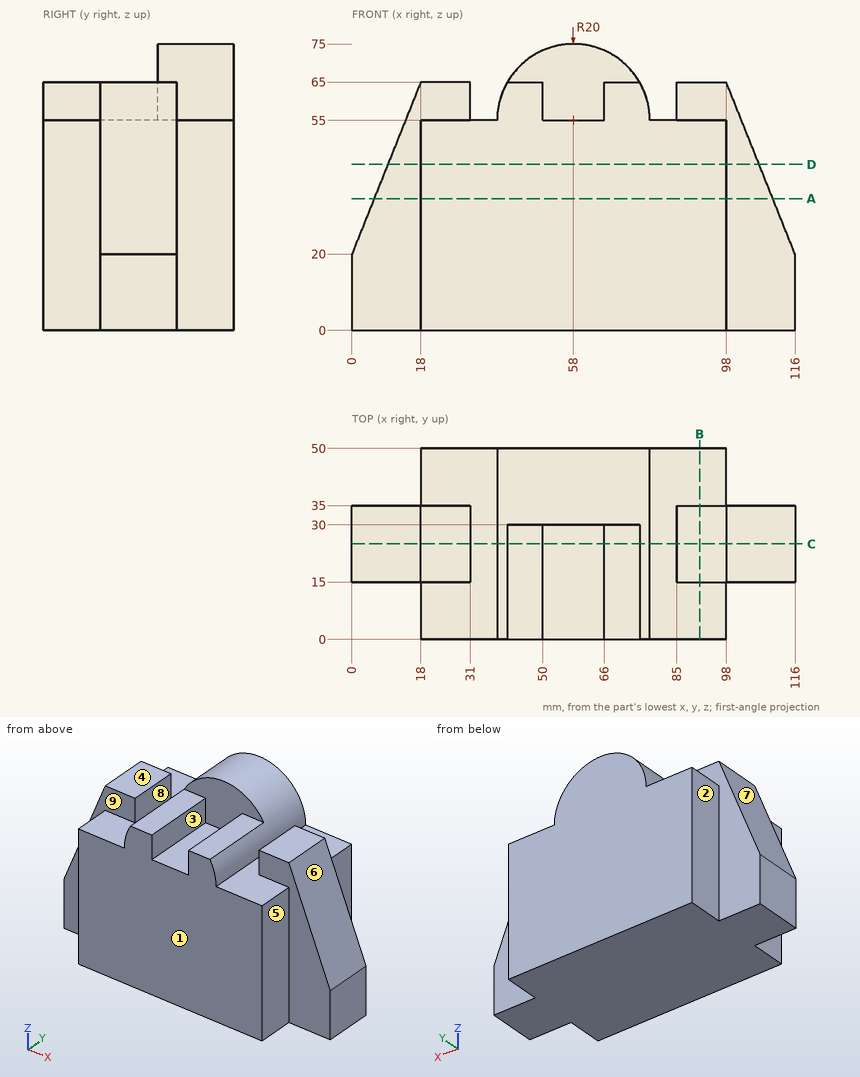
Could you check a few things on this drawing? It's one solid part, dimensions in mm from its lowest x, y, z. A direction names the side the tool comes from. Coordinates: 2 decimals unless noted, no trailing zeros. Write each loop counter-clockwise with the first axis right and the second up, starting at its lowest first coordinate (ties: lowest second). Pieces come first, ordered by that corner, then holes. Notation, with made-up numbers: (49.25, 31.25) - (67.25, 31.25) arc R8 ccw to (67.25, 41.25) - close; hole circle Ø7 at (89.5, 11). An arc over 180 degrees is marked (long way). Return JSON: item names as keys, results as strings. Group by question number.
Item 1: Which directions (+Z, -Z, +X, -X, +Y, -Y) give clear straight access to the entire face, cutting with the end or side of a thin tool? Please do the marked faces 1, 2, 3, 4 and 5.
Item 2: If we section it at B-B (x = 91): Write out the boundary of the cut face in (y, z), then the cut area to 3 significant figures.
Item 3: Please list where these lines run through material, in increasing order: probe 1 along X at (y, z) = (17.5, 64.5); probe 2 along X at (y, z) = (4, 32.5); probe 3 along Z at (x, y) = (56, 13.5).
Item 4: If we section it at D-D (z = 43.5): Write out the boundary of the cut face in (x, y), then the cut area to 3 significant figures.
Item 5: If we section it at A-A (z = 34.5): Write out the boundary of the cut face in (x, y).
Item 6: We'd pull the mould along X, two halves only. Please class the marked faces 6, 7, 8 and 9: pulls with the +X half, pulls with the -X half, needs draft (parallel to the pull), parting line crosses it, or undercut.
Item 7: If we section it at C-C (y = 25): Write out the boundary of the cut face in (x, z), then the cut area to 3 significant figures.
Item 8: I'm going to push flat-ended pins straight in: pin 1 Ø12 at (x, y) = (90.5, 29) entering from +Z; pin 2 Ø4 at (y, z) = (38.5, 27.5) entering from +X; pin 3 Ø5 at (y, z) = (20, 59.5) entering from -X. Where does each tip first touch, or does it pass through?
Return value:
{
 "1": {"face 1": "+Z, -Z, +X, -X, -Y", "face 2": "+Z, -Z, -X, +Y", "face 3": "+Z, -Y", "face 4": "+Z, -X, +Y, -Y", "face 5": "+Z, -Z, +X, -Y"},
 "2": {"outline": "(0, 0) - (50, 0) - (50, 55) - (35, 55) - (35, 65) - (15, 65) - (15, 55) - (0, 55) - close", "area": "2,950 mm^2"},
 "3": {"probe 1": "x = 17.8 to 31, 40.4 to 50, 66 to 75.6, 85 to 98.2", "probe 2": "x = 18 to 98", "probe 3": "z = 0 to 55"},
 "4": {"outline": "(9.4, 15) - (18, 15) - (18, 0) - (98, 0) - (98, 15) - (106.6, 15) - (106.6, 35) - (98, 35) - (98, 50) - (18, 50) - (18, 35) - (9.4, 35) - close", "area": "4,340 mm^2"},
 "5": {"outline": "(5.8, 15) - (18, 15) - (18, 0) - (98, 0) - (98, 15) - (110.2, 15) - (110.2, 35) - (98, 35) - (98, 50) - (18, 50) - (18, 35) - (5.8, 35) - close"},
 "6": {"face 6": "pulls with the +X half", "face 7": "pulls with the -X half", "face 8": "undercut", "face 9": "needs draft"},
 "7": {"outline": "(0, 0) - (116, 0) - (116, 20) - (98, 65) - (85, 65) - (85, 55) - (78, 55) arc R20 ccw to (75.32, 65) - (66, 65) - (66, 55) - (50, 55) - (50, 65) - (40.68, 65) arc R20 ccw to (38, 55) - (31, 55) - (31, 65) - (18, 65) - (0, 20) - close", "area": "6,410 mm^2"},
 "8": {"pin 1": "stops at z = 65", "pin 2": "stops at x = 98", "pin 3": "stops at x = 14.8"}
}
